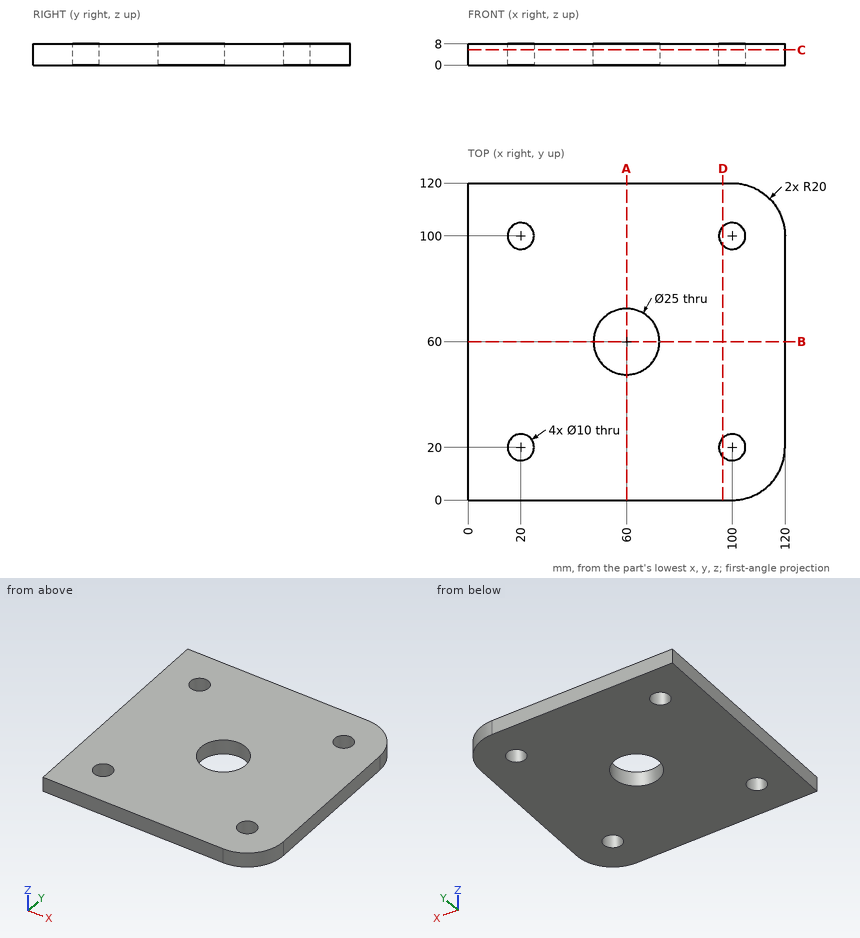
Could you check a few things on this drawing? It's one solid part, dimensions in mm from its lowest x, y, z. Coordinates: 2 decimals unless noted, no trailing zeros. Order: outer loops, then holes, each group sorted by start corner. A loop starts at its lowest first (then second) coordinate and runs counter-clockwise, first axis right, second up. Notation, with made-up numbers: (49.5, 50.5) -> (94.5, 50.5) arc R19 cw to (94.5, 81.5) -> close; hole circle Ø2 at (59.5, -1). An arc over 180 degrees is marked (long way). One line per item, written item: value. Start each with the question number.
1) I'm going to push a flat-ended pin straight in: pin 1 (9 mm diameter, centred on x = 20, y = 100, fed in from +Z). Where does the tip first touch, or does it pass through?
2) Imagine slicing it at A-A on x = 60. List the corners of the cut face in (y, z) for me, plus the area to 3 significant figures.
3) Imagine slicing it at D-D on x = 96.5. List the corners of the cut face in (y, z) for me, plus the area to 3 significant figures.
4) If I drill on L1, parallel to Y at x = 20, z = 5; L2, parallel to X at y = 96, z = 6.25; L3, parallel to X at y = 52, z = 6.25, over which ranges is the centre line in solid material (lowest first)? Write a range as [from, to].
5) Imagine slicing it at C-C on z = 5.75. List the corners of the cut face in (x, y) for me.
Answer list:
1. pin 1: passes through
2. outline: (0, 0) -> (47.5, 0) -> (47.5, 8) -> (0, 8) -> close; (72.5, 0) -> (120, 0) -> (120, 8) -> (72.5, 8) -> close
2. area: 760 mm2
3. outline: (0, 0) -> (16.43, 0) -> (16.43, 8) -> (0, 8) -> close; (23.57, 0) -> (96.43, 0) -> (96.43, 8) -> (23.57, 8) -> close; (103.57, 0) -> (120, 0) -> (120, 8) -> (103.57, 8) -> close
3. area: 846 mm2
4. L1: y = [0, 15], [25, 95], [105, 120]
4. L2: x = [0, 17], [23, 97], [103, 120]
4. L3: x = [0, 50.4], [69.6, 120]
5. outline: (0, 0) -> (100, 0) arc R20 ccw to (120, 20) -> (120, 100) arc R20 ccw to (100, 120) -> (0, 120) -> close; hole circle Ø10 at (20, 20); hole circle Ø10 at (20, 100); hole circle Ø25 at (60, 60); hole circle Ø10 at (100, 20); hole circle Ø10 at (100, 100)
